Job drawing, mm, ordinate dimensions from the low corner. One solid piece. Give positions to 0.01 mm unless a question says otherwise; leave off trailing zeros. Order: outer loops, then holes, each group sorted by start corner. A loop starts at its lowest first (then second) coordinate and runs counter-clockwise, first axis right, second up. Notation, with made-up numbers: M 4.25,-20.75 L 48.25,-20.75 A8 cw 48.25,-8.75 Z; hole C 26.25,-9.75 d2. An arc over 180 degrees is marked long. Put each result on its own line as item: value. Start each with the question number.
1) Cut at B-B (y = 8.25). Write the cut outline in (x, z).
2) Cut at A-A (x = 5). Write the cut outline in (y, z).
3) Drill centre lines: line 1 (Z direction, x = 21.25, y = 5); line 2 (Y direction, x = 4.5, z = 48.5). Where is each one in solid material? Low to high. Write a range as [from, to].
4) Pin check, flat tip, straight feed: pin 1 (8 mm diameter, centred on x = 9.5, y = 8.5, fed in from -Z). Stop position of the tip, or through.
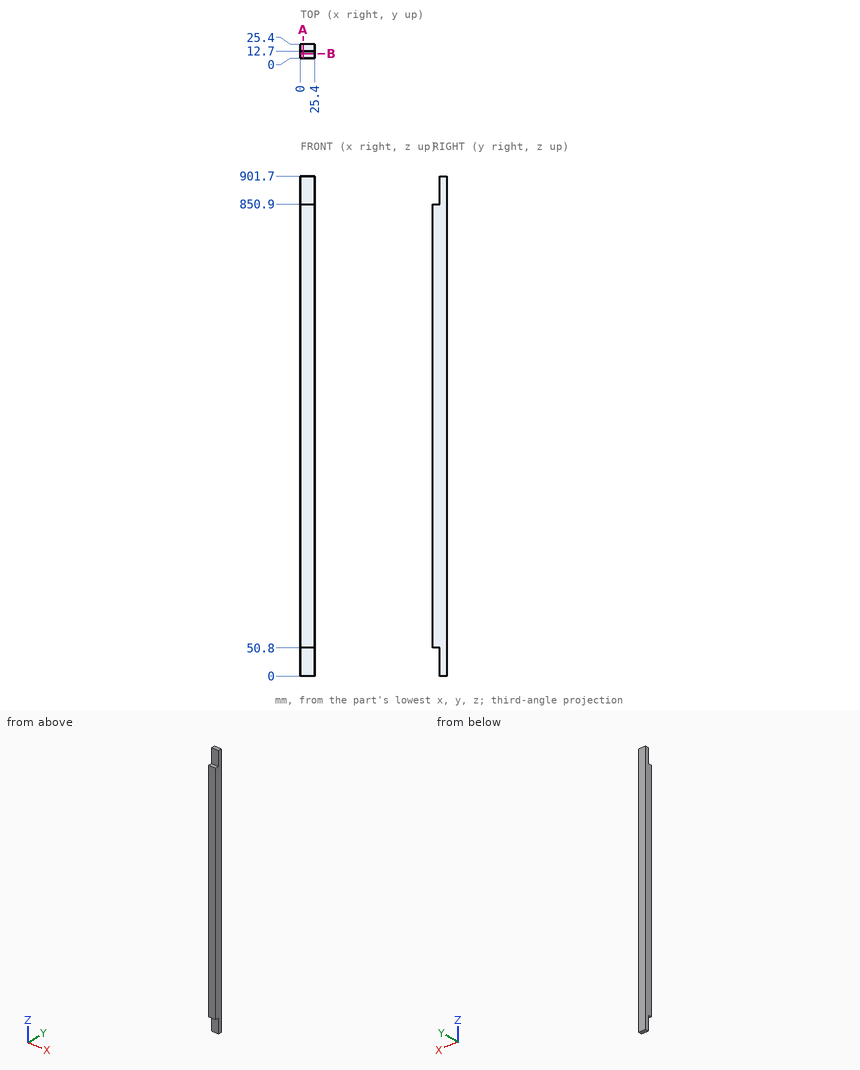
Solution:
1. outline: M 0,50.8 L 25.4,50.8 L 25.4,850.9 L 0,850.9 Z
2. outline: M 0,50.8 L 12.7,50.8 L 12.7,0 L 25.4,0 L 25.4,901.7 L 12.7,901.7 L 12.7,850.9 L 0,850.9 Z
3. line 1: [50.8, 850.9]
3. line 2: [12.7, 25.4]
4. pin 1: z = 50.8
